Work out the finished part from the listing and answer in its coordinate system (mm). Coordinates: 2 decimals unless noted, no trailing zeros. Loops run counter-clockwise (first coordinate to the right, second up) from the corner with the lowest first, then second, coordinate; pieces in that order, holes last. Notation, with made-up numbers: (29.25, 50) -> (75.25, 50) arc R20 cw to (75.25, 83) -> close; hole circle Ø3 at (21, 29). An arc over 180 degrees is marked (long way). Use a Markdown table: item, result. Add a question column.
```python
from build123d import *

# Parameters (mm, degrees)
SKETCH1_R                      = 79.375
BOSS_EXTRUDE1_DEPTH            = 3.175
SKETCH2_R                      = 76.2
BOSS_EXTRUDE2_DEPTH            = 3.175
F_1_4_0_25_DIAMETER_HOLE1_D    = 6.35
F_1_16_0_0625_DIAMETER_HOLE1_D = 1.5875
F_3_8_0_375_DIAMETER_HOLE1_D   = 9.525


with BuildPart() as part:
    # Sketch1 → Boss-Extrude1 (new body)
    with BuildSketch(Plane.XY):
        Circle(SKETCH1_R)
    extrude(amount=BOSS_EXTRUDE1_DEPTH)

    # Sketch2 → Boss-Extrude2 (add)
    with BuildSketch(Plane.XY.offset(3.175)):
        Circle(SKETCH2_R)
    extrude(amount=BOSS_EXTRUDE2_DEPTH)

    # 1/4 (0.25) Diameter Hole1 (through all)
    with Locations(Plane.XY.offset(6.35)):
        with Locations((-44.45, -9.525), (44.45, -9.525)):
            Hole(F_1_4_0_25_DIAMETER_HOLE1_D / 2)

    # 1/16 (0.0625) Diameter Hole1 (through all)
    with Locations(Plane.XY.offset(6.35)):
        with Locations((-19.05, 44.45), (-6.35, 44.45), (6.35, 44.45), (19.05, 44.45)):
            Hole(F_1_16_0_0625_DIAMETER_HOLE1_D / 2)

    # 3/8 (0.375) Diameter Hole1 (through all)
    with Locations(Plane.XY.offset(6.35)):
        with Locations((0, -26.9875), (0, 26.9875)):
            Hole(F_3_8_0_375_DIAMETER_HOLE1_D / 2)


solid = part.part
```
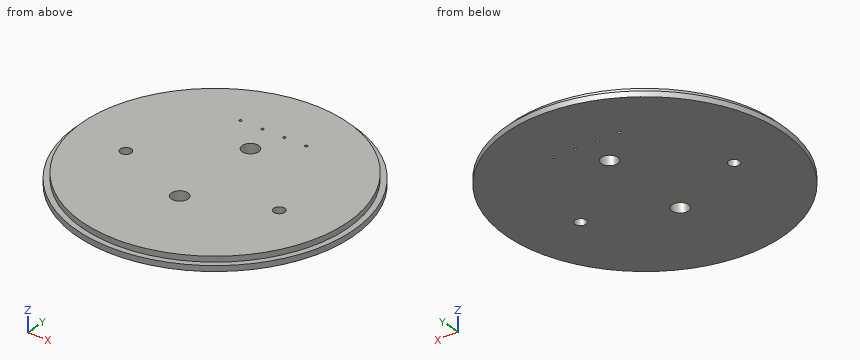
Item 1: Section B-B (z = 1) is taken. Count the separate pieces of the cut face and the enclosed holes in it, then the cut area to 3 significant figures.
Item 2: Section A-A (x = 0) is taken. Determine the outline of the cut face in (y, z) (3 decimals).
Item 3: Given pin 1 (1.5 mm diameter, centred on y = 12.5, z = 3.5, fed in from -X); pin 2 (3 mm diameter, centred on x = 60, z = 1, fed in from +Y); pin 3 (2 mm diameter, centred on y = -50, z = 2, fed in from +X), each flat-ended and moving along its own axis, determine where each tip first touches the part or whether it passes through.
Item 4: Find the intervals of material crossed by probe 1 along Y at (x, z) = (0, 5.25) (3 decimals); probe 2 along X at (y, z) = (44.45, 2.75); probe 3 along Y at (x, z) = (-44.45, 2.5), in increasing order.
Item 5: Section D-D (y = 0) is taken. Determine the outline of the cut face in (x, z) (3 decimals).
Item 6: Section C-C (x = -44.45) is taken. Determine the outline of the cut face in (y, z) (3 decimals).
Output:
| question | item | result |
|---|---|---|
| 1 | separate pieces | 1 |
| 1 | enclosed holes | 8 |
| 1 | area | 19,600 mm2 |
| 2 | outline | (-79.375, 0) -> (-31.75, 0) -> (-31.75, 6.35) -> (-76.2, 6.35) -> (-76.2, 3.175) -> (-79.375, 3.175) -> close; (-22.225, 0) -> (22.225, 0) -> (22.225, 6.35) -> (-22.225, 6.35) -> close; (31.75, 0) -> (79.375, 0) -> (79.375, 3.175) -> (76.2, 3.175) -> (76.2, 6.35) -> (31.75, 6.35) -> close |
| 3 | pin 1 | stops at x = -78.49 |
| 3 | pin 2 | stops at y = 53.65 |
| 3 | pin 3 | stops at x = 62.45 |
| 4 | probe 1 | y = -76.2 to -31.75, -22.225 to 22.225, 31.75 to 76.2 |
| 4 | probe 2 | x = -65.76 to -19.84, -18.26 to -7.14, -5.56 to 5.56, 7.14 to 18.26, 19.84 to 65.76 |
| 4 | probe 3 | y = -65.76 to -12.7, -6.35 to 65.76 |
| 5 | outline | (-79.375, 0) -> (79.375, 0) -> (79.375, 3.175) -> (76.2, 3.175) -> (76.2, 6.35) -> (-76.2, 6.35) -> (-76.2, 3.175) -> (-79.375, 3.175) -> close |
| 6 | outline | (-65.762, 0) -> (-12.7, 0) -> (-12.7, 6.35) -> (-61.892, 6.35) -> (-61.892, 3.175) -> (-65.762, 3.175) -> close; (-6.35, 0) -> (65.762, 0) -> (65.762, 3.175) -> (61.892, 3.175) -> (61.892, 6.35) -> (-6.35, 6.35) -> close |
